Part model, mm, in its own coordinate system. Face numbers are marked on the shaded views. Coordinates: 2 decimals unless noted, no trailing zeros. Loops run counter-clockwise (first coordinate to the right, second up) from the corner with the lowest first, then second, coordinate; pieces in that order, holes last. Notation, with made-up numbers: M 13,48 L 32,48 A32 ccw 32,86 Z; hole C -18,-2 d1. An arc over 180 degrees is marked long. Use a Markdown table: item, result. Add a question column.
1) Band-saw the part on A-A (x = 0). List the corners of the cut face in (y, z), plus the area to 3 significant figures.
2) Pull direction Z, two halves, no side cores. Call the marked faces 1, 2, 3 and 4: released by +Z, released by -Z, zero draft, split by the parting line, or undercut.
3) Band-saw the part on C-C (y = 5.5). List the corners of the cut face in (x, z).
4) Wall check: probe 1 along Z at (x, y) = (0, 37); probe 2 along X at (y, z) = (3.25, 19.05); probe 3 along X at (y, z) = (31, 8.5). Give the ranges that are in metal, low to high. Write a range as from..to.
5) Pin check, flat tips, straight feed: pin 1 Ø3 at (x, z) = (-7.5, 27.5) entering from +Y; pin 2 Ø7.5 at (x, z) = (0, 19.05) entering from +Y; pin 3 Ø2 at (y, z) = (26, 16.5) entering from +X; pin 4 Ø3 at (x, z) = (-5.5, 15.5) entering from +Y. Stop position of each tip, or through.
6) Band-saw the part on B-B (z = 19.05). List the corners of the cut face in (x, y).
7) Band-saw the part on D-D (x = -8). List the corners of the cut face in (y, z), plus the area to 3 significant figures.
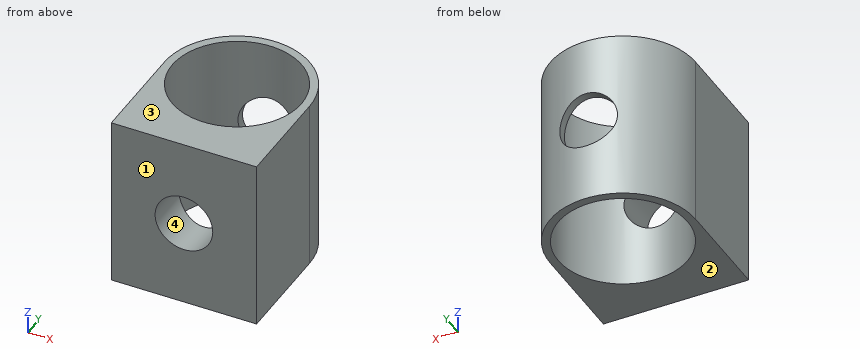
from build123d import *

# Parameters (mm, degrees)
SKETCH1_R           = 14.224
BOSS_EXTRUDE1_DEPTH = 38.1
SKETCH2_R           = 6.35
CUT_EXTRUDE1_DEPTH  = 39.7096


with BuildPart() as part:
    # Sketch1 → Boss-Extrude1 (new body)
    with BuildSketch(Plane.XY):
        with BuildLine():
            Line((16, 0), (-16, 0))
            Line((-16, 0), (-16, 22.7096))
            ThreePointArc((-16, 22.7096), (0, 38.7096), (16, 22.7096))
            Line((16, 22.7096), (16, 0))
        make_face()
        with Locations((0, 22.7096)):
            Circle(SKETCH1_R, mode=Mode.SUBTRACT)
    extrude(amount=BOSS_EXTRUDE1_DEPTH)

    # Sketch2 → Cut-Extrude1 (cut, through all)
    with BuildSketch(Plane.XZ):
        with Locations((0, 19.05)):
            Circle(SKETCH2_R)
    extrude(amount=-CUT_EXTRUDE1_DEPTH, mode=Mode.SUBTRACT)


solid = part.part
Entries:
| question | item | result |
|---|---|---|
| 1 | outline | M 0,0 L 8.49,0 L 8.49,12.7 L 0,12.7 Z; M 0,25.4 L 8.49,25.4 L 8.49,38.1 L 0,38.1 Z; M 36.93,0 L 38.71,0 L 38.71,12.7 L 36.93,12.7 Z; M 36.93,25.4 L 38.71,25.4 L 38.71,38.1 L 36.93,38.1 Z |
| 1 | area | 261 mm2 |
| 2 | face 1 | zero draft |
| 2 | face 2 | released by -Z |
| 2 | face 3 | released by +Z |
| 2 | face 4 | undercut |
| 3 | outline | M -16,0 L 16,0 L 16,38.1 L -16,38.1 Z; hole C 0,19.05 d12.7 |
| 4 | probe 1 | 0..12.7, 25.4..38.1 |
| 4 | probe 2 | -16..-6.35, 6.35..16 |
| 4 | probe 3 | -13.68..-11.56, 11.56..13.68 |
| 5 | pin 1 | y = 37.54 |
| 5 | pin 2 | through |
| 5 | pin 3 | x = 15.84 |
| 5 | pin 4 | y = 38.09 |
| 6 | outline | M -16,0 L -6.35,0 L -6.35,9.98 A14.22 cw -6.35,35.44 L -6.35,37.4 A16 ccw -16,22.71 Z; M 6.35,0 L 16,0 L 16,22.71 A16 ccw 6.35,37.4 L 6.35,35.44 A14.22 cw 6.35,9.98 Z |
| 7 | outline | M 0,0 L 10.95,0 L 10.95,38.1 L 0,38.1 Z; M 34.47,0 L 36.57,0 L 36.57,38.1 L 34.47,38.1 Z |
| 7 | area | 497 mm2 |
